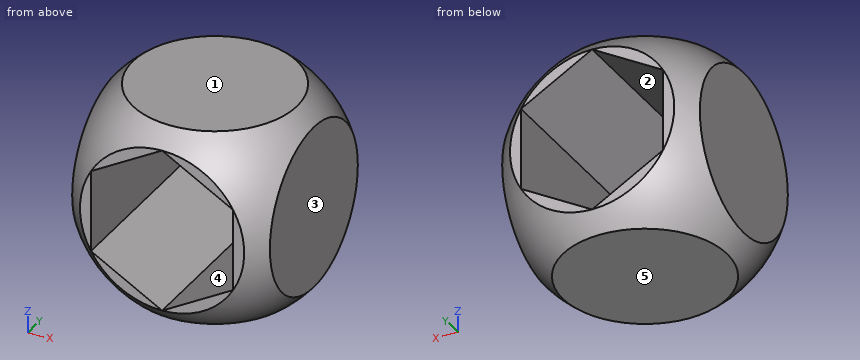
```python
from build123d import *

# Parameters (mm, degrees)
P_IDAT_VYSUNUT_M1_DEPTH      = 50
P_IDAT_VYSUNUT_M1_DEPTH_BACK = 50
SKICA2_W                     = 100
SKICA2_H                     = 100
ODEBRAT_VYSUNUT_M1_DEPTH     = 123.474487139


with BuildPart() as part:
    # Skica1 → Rotovat1 (revolve)
    with BuildSketch(Plane.XY):
        with BuildLine():
            Line((0, 0), (-65, 0))
            ThreePointArc((-65, 0), (0, 65), (65, 0))
            Line((65, 0), (0, 0))
        make_face()
    revolve(axis=Axis((0, 0, 0), (1, 0, 0)))


with BuildPart() as body_2:
    # Skica2 → Přidat vysunutím1 (new, two sides: drawn at the far end of the back side and taken through both)
    with BuildSketch(Plane.XY.offset(-P_IDAT_VYSUNUT_M1_DEPTH_BACK)):
        Rectangle(SKICA2_W, SKICA2_H)
    extrude(amount=P_IDAT_VYSUNUT_M1_DEPTH + P_IDAT_VYSUNUT_M1_DEPTH_BACK)


with BuildPart() as part_1:
    add(part.part)

    # Průsečík1: read off the stored shape, not the designer's step
    # Průsečík1: intersect body 2
    add(body_2.part, mode=Mode.INTERSECT)

    # Skica3 → Odebrat vysunutím1 (cut, through all)
    with BuildSketch(Plane(origin=(0, 50, 0), x_dir=(1, 0, 0), z_dir=(0, 1, 0))):
        Polygon((0, 41.533119315), (-35.968736425, 20.766559657), (-35.968736425, -20.766559657), (0, -41.533119315), (35.968736425, -20.766559657), (35.968736425, 20.766559657), align=None)
    extrude(amount=-ODEBRAT_VYSUNUT_M1_DEPTH, mode=Mode.SUBTRACT)


solid = part_1.part
```
Model file for the job. Use its own axes, mm. Face numbers are marked on the shaded views. A direction names the side the tool comes from. Give positions to 0.01 mm unless a question says otherwise; leave off trailing zeros. Loops run counter-clockwise (first coordinate to the right, second up) from the corner with the lowest first, then second, coordinate; pieces in that order, holes last. Notation, with made-up numbers: (87, 81) -> (93, 81) arc R23 cw to (93, 95) -> close; hole circle Ø7 at (2.5, -4.5). An arc over 180 degrees is marked (long way). Use CSV: the item, a comma, the result in double quotes. Start each with the question number.
1) Slice it at B-B on y = -39.5. Give the cut face in (x, z).
2) Slice it at C-C on z = 17.5. Give the cut face in (x, y).
3) Slice it at D-D on y = -18.5. Give the cut face in (x, z).
4) Tool access for the marked faces 4 and 5: list every direction of +Z, -Z, +X, -X, +Y, -Y with a clear straight run to the whole face (end or side of a thin tool).
5) Mould opens along X. For the marked faces 1, 2 and 3 say: released by +X, released by -X, zero draft, split by the parting line, or undercut.
6) Slice it at A-A on x = 21. Give the cut face in (y, z), plus the area to 3 significant figures.
7) Wall check: line 1 (X direction, y = 35, z = -3.5); line 2 (Z direction, x = 14, y = -14); line 3 (Z direction, x = -34, y = -0.5). Give the ranges that are in metal, low to high.
Computed values:
1,outline,"(-50, -12.84) arc R51.62 ccw to (-12.84, -50) -> (12.84, -50) arc R51.62 ccw to (50, -12.84) -> (50, 12.84) arc R51.62 ccw to (12.84, 50) -> (-12.84, 50) arc R51.62 ccw to (-50, 12.84) -> close; hole (-35.97, -20.77) -> (0, -41.53) -> (35.97, -20.77) -> (35.97, 20.77) -> (0, 41.53) -> (-35.97, 20.77) -> close"
2,outline,"(-50, -37.67) arc R62.6 ccw to (-37.67, -50) -> (-35.97, -50) -> (-35.97, 50) -> (-37.67, 50) arc R62.6 ccw to (-50, 37.67) -> close; (35.97, -50) -> (37.67, -50) arc R62.6 ccw to (50, -37.67) -> (50, 37.67) arc R62.6 ccw to (37.67, 50) -> (35.97, 50) -> close"
3,outline,"(-50, -37.19) arc R62.31 ccw to (-37.19, -50) -> (37.19, -50) arc R62.31 ccw to (50, -37.19) -> (50, 37.19) arc R62.31 ccw to (37.19, 50) -> (-37.19, 50) arc R62.31 ccw to (-50, 37.19) -> close; hole (-35.97, -20.77) -> (0, -41.53) -> (35.97, -20.77) -> (35.97, 20.77) -> (0, 41.53) -> (-35.97, 20.77) -> close"
4,face 4,"+Y, -Y"
4,face 5,"-Z, +X, -X, +Y, -Y"
5,face 1,"zero draft"
5,face 2,"undercut"
5,face 3,"released by +X"
6,outline,"(-50, -35.83) arc R61.51 ccw to (-35.83, -50) -> (35.83, -50) arc R61.51 ccw to (50, -35.83) -> (50, -29.41) -> (-50, -29.41) -> close; (-50, 29.41) -> (50, 29.41) -> (50, 35.83) arc R61.51 ccw to (35.83, 50) -> (-35.83, 50) arc R61.51 ccw to (-50, 35.83) -> close"
6,area,"3,760 mm^2"
7,line 1,"x = -50 to -35.97, 35.97 to 50"
7,line 2,"z = -50 to -33.45, 33.45 to 50"
7,line 3,"z = -50 to -21.9, 21.9 to 50"
